For this review, take the finished solid that the model builds, in its own axes (mm). A direction names the side the tool comes from. Give positions to 0.01 mm unless a question says otherwise; leave off trailing zeros. Order: outer loops, then holes, each group sorted by start corner. A loop starts at its lowest first (then second) coordinate and runs counter-clockwise, first axis right, second up. Notation, with made-up numbers: (7, 40.5) - (12, 40.5) arc R35 ccw to (12, 79.5) - close; hole circle Ø7 at (23.5, 84). An arc over 180 degrees is marked (long way). Use a Markdown table: item, result. Add a question column.
1) We need section B-B on x = 179. Write out the cut boundary in (y, z) (3 decimals), then the cut area to 3 significant figures.
2) We need section C-C on z = 455. Write out the cut boundary in (x, y) (3 decimals).
3) Machinability: for faces 1 (the face through (297, -28.575, 319)), 2 (the face through (314.96, -16, 313)), which of the approach directions +Z, -Z, +X, -X, +Y, -Y give a long, thin tool a straight path to every point of the face, cutting with its end or side? Answer none if there is none.
4) Wall thickness on L1, parallel to X at y = -15.5, z = 573.5; L2, parallel to Z at x = 1053, y = -20; L3, parallel to Y at x = 711.5, z = 186 (3 decimals): over which ranges is each line inside the solid? List them lowest first.
5) We need section A-A on y = -11.25. Write out the cut boundary in (x, z), then the cut area to 3 significant figures.
6) Mouldability with a two-part tool opening along Z and no side actions: class faces 3 (the face through (726, -14, 0)), 4 (the face through (0, -14, 322)), 5 (the face through (735, -16, 609.6)) as released by +Z, released by -Z, zero draft, split by the parting line, or undercut.
7) Clearance check with flat-ended pins moving along their axes: P1, Ø12.5, axis at x = 1064, y = -12, coming from the -Z side; P2, Ø8, axis at x = 425, z = 237.5, coming from the -Y side (3 decimals). State where each tip first meets the part, or that it passes through.
```python
from build123d import *

# Parameters (mm, degrees)
F0_W     = 1473.2
F0_H     = 635
F1_DEPTH = 3.175
F2_W     = 25.4
F2_H     = 584.2
F3_DEPTH = 25.4


with BuildPart() as f1:
    # F0 (on Front) → F1 (new body)
    with BuildSketch(Plane.XZ):
        with Locations((736.6, 317.5)):
            Rectangle(F0_W, F0_H)
    extrude(amount=F1_DEPTH)

    # F2 (on face) → F3 (join)
    with BuildSketch(Plane.XZ.offset(3.175)):
        Polygon((0, 25.4), (0, 0), (1473.2, 0), (1473.2, 25.4), (1447.8, 25.4), (1183.64, 25.4), (1158.24, 25.4), (894.08, 25.4), (868.68, 25.4), (604.52, 25.4), (579.12, 25.4), (314.96, 25.4), (289.56, 25.4), (25.4, 25.4), align=None)
        with Locations((12.7, 317.5)):
            Rectangle(F2_W, F2_H)
        with Locations((1460.5, 317.5)):
            Rectangle(F2_W, F2_H)
        Polygon((0, 635), (0, 609.6), (25.4, 609.6), (289.56, 609.6), (314.96, 609.6), (579.12, 609.6), (604.52, 609.6), (868.68, 609.6), (894.08, 609.6), (1158.24, 609.6), (1183.64, 609.6), (1447.8, 609.6), (1473.2, 609.6), (1473.2, 635), align=None)
        with Locations((302.26, 317.5)):
            Rectangle(F2_W, F2_H)
        with Locations((591.82, 317.5)):
            Rectangle(F2_W, F2_H)
        with Locations((881.38, 317.5)):
            Rectangle(F2_W, F2_H)
        with Locations((1170.94, 317.5)):
            Rectangle(F2_W, F2_H)
    extrude(amount=F3_DEPTH)


solid = f1.part
```
Checked values:
| question | item | result |
|---|---|---|
| 1 | outline | (-28.575, 0) - (0, 0) - (0, 635) - (-28.575, 635) - (-28.575, 609.6) - (-3.175, 609.6) - (-3.175, 25.4) - (-28.575, 25.4) - close |
| 1 | area | 3,310 mm² |
| 2 | outline | (0, -28.575) - (25.4, -28.575) - (25.4, -3.175) - (289.56, -3.175) - (289.56, -28.575) - (314.96, -28.575) - (314.96, -3.175) - (579.12, -3.175) - (579.12, -28.575) - (604.52, -28.575) - (604.52, -3.175) - (868.68, -3.175) - (868.68, -28.575) - (894.08, -28.575) - (894.08, -3.175) - (1158.24, -3.175) - (1158.24, -28.575) - (1183.64, -28.575) - (1183.64, -3.175) - (1447.8, -3.175) - (1447.8, -28.575) - (1473.2, -28.575) - (1473.2, 0) - (0, 0) - close |
| 3 | face 1 | +Z, -Z, +X, -X, -Y |
| 3 | face 2 | -Y |
| 4 | L1 | 0 to 25.4, 289.56 to 314.96, 579.12 to 604.52, 868.68 to 894.08, 1158.24 to 1183.64, 1447.8 to 1473.2 |
| 4 | L2 | 0 to 25.4, 609.6 to 635 |
| 4 | L3 | -3.175 to 0 |
| 5 | outline | (0, 0) - (1473.2, 0) - (1473.2, 635) - (0, 635) - close; hole (25.4, 25.4) - (289.56, 25.4) - (289.56, 609.6) - (25.4, 609.6) - close; hole (314.96, 25.4) - (579.12, 25.4) - (579.12, 609.6) - (314.96, 609.6) - close; hole (604.52, 25.4) - (868.68, 25.4) - (868.68, 609.6) - (604.52, 609.6) - close; hole (894.08, 25.4) - (1158.24, 25.4) - (1158.24, 609.6) - (894.08, 609.6) - close; hole (1183.64, 25.4) - (1447.8, 25.4) - (1447.8, 609.6) - (1183.64, 609.6) - close |
| 5 | area | 164,000 mm² |
| 6 | face 3 | released by -Z |
| 6 | face 4 | zero draft |
| 6 | face 5 | undercut |
| 7 | P1 | z = 0 |
| 7 | P2 | y = -3.175 |
